Source: CAD feature listing. Evaluate the final solid. Frame: model axes, mm. A direction names the side the tool comes from. Give positions to 0.01 mm unless a question says otherwise; leave off trailing zeros. Write each loop counter-clockwise with the first axis right and the second up, starting at its lowest first coordinate (ties: lowest second). Pieces come first, ordered by that corner, then holes. Notation, with made-up numbers: M 21.25,24 L 56.25,24 A21 ccw 56.25,35 Z; hole C 85.5,87 d5. An arc over 180 degrees is marked long. Return JSON: item names as keys, results as strings.
```python
from build123d import *

# Parameters (mm, degrees)
BOSS_EXTRUDE1_DEPTH      = 20
BOSS_EXTRUDE1_DEPTH_BACK = 20
SKETCH4_W                = 10.912387574
SKETCH4_H                = 53.553398504
CUT_EXTRUDE1_DEPTH       = 10
CUT_EXTRUDE1_DEPTH_BACK  = 10
BOSS_EXTRUDE2_DEPTH      = 10
BOSS_EXTRUDE2_DEPTH_BACK = 10


with BuildPart() as part:
    # Sketch2 → Boss-Extrude1 (new body, two sides)
    with BuildSketch(Plane.XY) as boss_extrude1_sk:
        with BuildLine():
            Line((0, -35.697454944), (0, 35.697454944))
            Line((0, 35.697454944), (6.009448328, 35.697454944))
            add(Edge.make_bspline(
                [(6.009448328, 35.697454944), (10.056825281, 0), (6.009448328, -35.697454944)],
                knots=[0, 0, 0, 1, 1, 1], degree=2))
            Line((6.009448328, -35.697454944), (0, -35.697454944))
        make_face()
    extrude(amount=BOSS_EXTRUDE1_DEPTH)
    extrude(boss_extrude1_sk.sketch, amount=-BOSS_EXTRUDE1_DEPTH_BACK)

    # Sketch4 → Cut-Extrude1 (cut, two sides)
    with BuildSketch(Plane.XY) as cut_extrude1_sk:
        with Locations((10.034480552, 1.197125595)):
            Rectangle(SKETCH4_W, SKETCH4_H)
    extrude(amount=CUT_EXTRUDE1_DEPTH, mode=Mode.SUBTRACT)
    extrude(cut_extrude1_sk.sketch, amount=-CUT_EXTRUDE1_DEPTH_BACK, mode=Mode.SUBTRACT)

    # Sketch3 → Boss-Extrude2 (add, two sides)
    with BuildSketch(Plane.XY) as boss_extrude2_sk:
        Polygon((4.578286765, 27.973824847), (4.578286765, -25.579573657), (15.490674339, -25.579573657), align=None)
    extrude(amount=BOSS_EXTRUDE2_DEPTH)
    extrude(boss_extrude2_sk.sketch, amount=-BOSS_EXTRUDE2_DEPTH_BACK)


solid = part.part
```
1) Contact query for flat-ended pins moving along their axis: pin 1 Ø3 at (y, z) = (27.5, 14.5) entering from -X; pin 2 Ø7 at (x, y) = (13.5, 0.5) entering from +Z; pin 3 Ø2.5 at (x, z) = (10, 1.5) entering from -Y; pin 4 Ø8 at (y, z) = (16, 6) entering from +X. Output: stop coordinate, or through.
Numbers:
{"pin 1": "stops at x = 0", "pin 2": "stops at z = 10", "pin 3": "stops at y = -25.58", "pin 4": "stops at x = 7.83"}
2) Cut plane B-B, the plane x = 14.5. Return the cut outline in (y, z), then the cut area to 3 significant figures.
Numbers:
{"outline": "M -25.58,-10 L -20.72,-10 L -20.72,10 L -25.58,10 Z", "area": "97.2 mm²"}
3) Line query: line 1 (X direction, y = 2.5, z = -8.5); line 2 (X direction, y = -16, z = 2.5); line 3 (Z direction, x = 9.75, y = -3). Output: solid intervals per line, ascending. Write a range as [from, to].
Numbers:
{"line 1": "x = [0, 9.77]", "line 2": "x = [0, 13.54]", "line 3": "z = [-10, 10]"}
4) Draft query along Z for faces 1 (the face through (7, 23, 10)), 2 (the face through (10, -15, -10)), 3 (the face through (10, -15, 10)). Return one class per face: released by +Z, released by -Z, zero draft, split by the parting line, or undercut.
Numbers:
{"face 1": "undercut", "face 2": "released by -Z", "face 3": "released by +Z"}
5) Cut plane A-A, the plane x = 9.5. Return the cut outline in (y, z).
Numbers:
{"outline": "M -25.58,-10 L 3.82,-10 L 3.82,10 L -25.58,10 Z"}
6) Set-up query: faces 4 (the face through (7, 23, -10)), 5 (the face through (3, 35.697, 0)), 6 (the face through (11, -25.58, 0)). Return all of +Z, -Z, +X, -X, +Y, -Y with unobstructed straight access to the full face (end or side cutting, diameter ignored); none if empty.
Numbers:
{"face 4": "+X", "face 5": "+Z, -Z, +X, -X, +Y", "face 6": "+Z, -Z, +X, -Y"}
